Could you check a few things on this drawing? It's one solid part, dimensions in mm from its lowest x, y, z. A direction names the side the tool comes from. Give positions to 0.01 mm unless a question says otherwise; leave off trailing zeros. Loops run counter-clockwise (first coordinate to the right, second up) from the corner with the lowest first, then second, coordinate; pieces in that order, holes last. Notation, with made-up numbers: M 15,-3 L 19,-3 A33 ccw 19,32 Z; hole C 49,14 d9. An arc over 180 degrees is marked long. Answer in a Markdown table with one row per item. Add a question column.
1. I need wall thicknesses on line 1 along Y through (x, z) = (63.5, 5.25); line 2 along Z through (x, y) = (29, 47.5) (3 decimals); line 3 along Y through (x, z) = (107.95, 6.5). Which ranges of each line are inside material? Lowest first, please. Write a range as from..to.
2. If we section it at A-A on x = 63.5: List the corners of the cut face in (y, z) for me (3 decimals), then the cut area to 3 significant figures.
3. If we section it at C-C on z = 8: List the corners of the cut face in (x, y) for me, then the cut area to 3 significant figures.
4. If we section it at B-B on y = 50.8: List the corners of the cut face in (x, z) for me (3 decimals), then the cut area to 3 significant figures.
5. I'm going to push flat-ended pins straight in: pin 1 Ø12 at (x, y) = (101.5, 47.5) entering from +Z (3 decimals); pin 2 Ø1.5 at (y, z) = (76.5, 15) entering from +X. Where does each tip first touch, or does it pass through?
6. Which directions (+Z, -Z, +X, -X, +Y, -Y) give clear straight access to the entire face, cutting with the end or side of a thin tool? Please do the marked faces 1 and 2.
7. If we section it at D-D on y = 95.25: List the corners of the cut face in (x, z) for me (3 decimals), then the cut area to 3 significant figures.
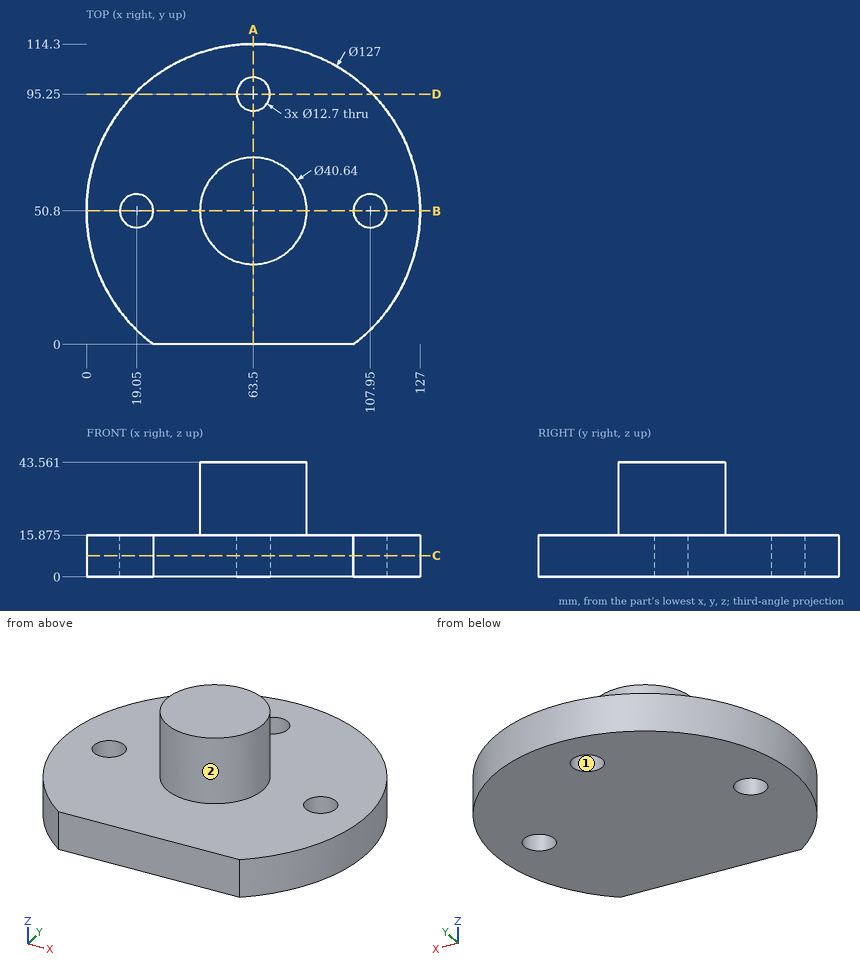
Results:
| question | item | result |
|---|---|---|
| 1 | line 1 | 0..88.9, 101.6..114.3 |
| 1 | line 2 | 0..15.875 |
| 1 | line 3 | 5.45..44.45, 57.15..96.15 |
| 2 | outline | M 0,0 L 88.9,0 L 88.9,15.875 L 71.12,15.875 L 71.12,43.561 L 30.48,43.561 L 30.48,15.875 L 0,15.875 Z; M 101.6,0 L 114.3,0 L 114.3,15.875 L 101.6,15.875 Z |
| 2 | area | 2,740 mm2 |
| 3 | outline | M 25.4,0 L 101.6,0 A63.5 ccw long Z; hole C 19.05,50.8 d12.7; hole C 63.5,95.25 d12.7; hole C 107.95,50.8 d12.7 |
| 3 | area | 11,600 mm2 |
| 4 | outline | M 0,0 L 12.7,0 L 12.7,15.875 L 0,15.875 Z; M 25.4,0 L 101.6,0 L 101.6,15.875 L 83.82,15.875 L 83.82,43.561 L 43.18,43.561 L 43.18,15.875 L 25.4,15.875 Z; M 114.3,0 L 127,0 L 127,15.875 L 114.3,15.875 Z |
| 4 | area | 2,740 mm2 |
| 5 | pin 1 | z = 15.875 |
| 5 | pin 2 | x = 121.89 |
| 6 | face 1 | +Z, -Z |
| 6 | face 2 | +Z |
| 7 | outline | M 18.152,0 L 57.15,0 L 57.15,15.875 L 18.152,15.875 Z; M 69.85,0 L 108.848,0 L 108.848,15.875 L 69.85,15.875 Z |
| 7 | area | 1,240 mm2 |
